Verification items for this drawing (mm, ordinates from the low corner). A direction names the side the tool comes from. Coordinates: 2 decimals unless noted, no trailing zeros. Write each loop counter-clockwise with the first axis right and the second up, starting at its lowest first coordinate (ties: lowest second). Pieces come first, ordered by that corner, then holes. Notation, with made-up numbers: (21.25, 66) -> (34.25, 66) arc R6 cw to (34.25, 70) -> close; hole circle Ø3 at (55, -7.5). An arc over 180 degrees is marked (long way). Answer as CSV lines item,"result".
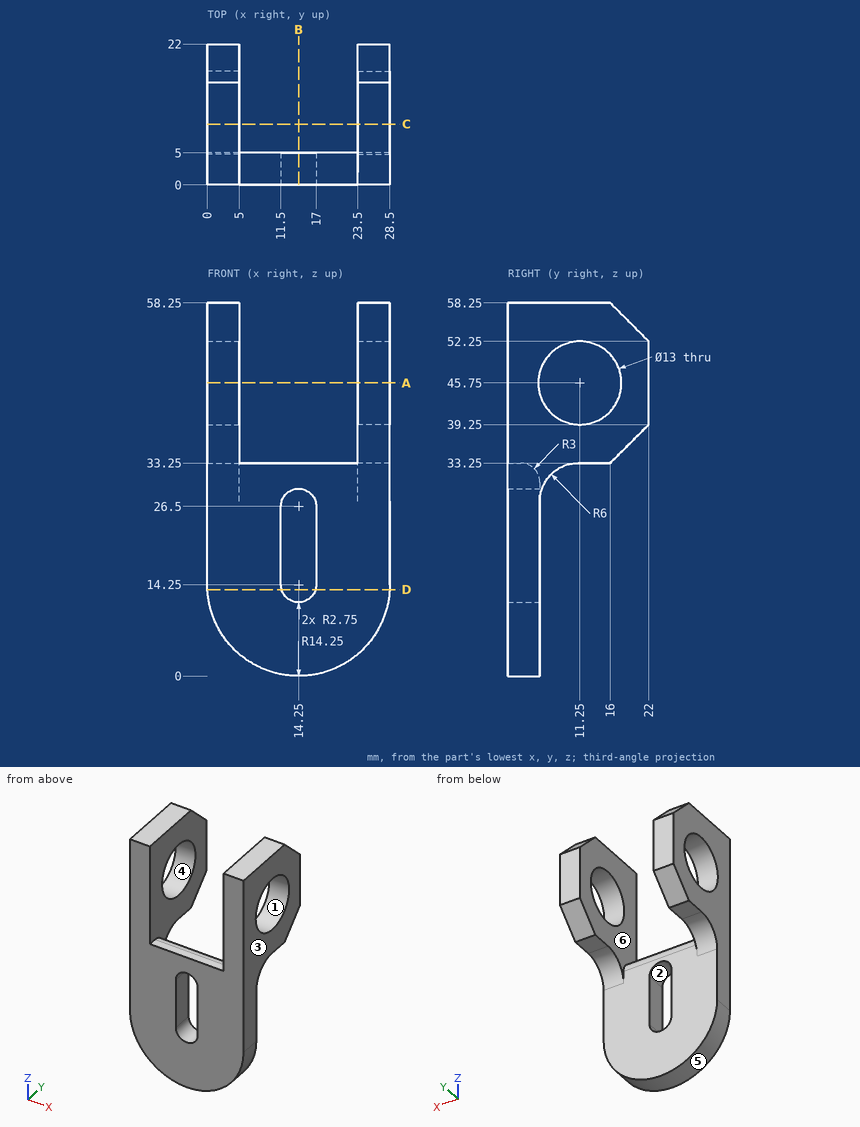
Item 1: Depth check by flat-ended pin: pin 1 Ø12 at (x, z) = (16.5, 7) entering from -Y; pin 2 Ø2 at (x, y) = (17, 0.5) entering from +Z; pin 3 Ø2.5 at (x, y) = (3, 14.5) entering from -Z; pin 4 Ø14 at (x, z) = (11, 22) entering from +Y. Enter the tip coordinate at first touch or a pass-through.
Responses:
pin 1,"stops at y = 0"
pin 2,"stops at z = 33.25"
pin 3,"stops at z = 33.25"
pin 4,"stops at y = 5"
Item 2: Set-up check for the marked faces 1 and 2: record each of +Z, -Z, +X, -X, +Y, -Y from which the full face is reachable in a straight line by a thin tool's end or side.
Responses:
face 1,"+X, -X"
face 2,"+Y, -Y"
Item 3: Cross-section at D-D, the plane z = 13.5. Record the cut outline in (x, y), plus the area to 3 significant figures.
Responses:
outline,"(0.02, 0) -> (11.6, 0) -> (11.6, 5) -> (0.02, 5) -> close; (16.9, 0) -> (28.48, 0) -> (28.48, 5) -> (16.9, 5) -> close"
area,"116 mm2"
Item 4: Cross-section at C-C, the plane y = 9.5. Record the cut outline in (x, z), plus the area to 3 significant figures.
Responses:
outline,"(0, 33.06) -> (5, 33.06) -> (5, 39.49) -> (0, 39.49) -> close; (0, 52.01) -> (5, 52.01) -> (5, 58.25) -> (0, 58.25) -> close; (23.5, 33.06) -> (28.5, 33.06) -> (28.5, 39.49) -> (23.5, 39.49) -> close; (23.5, 52.01) -> (28.5, 52.01) -> (28.5, 58.25) -> (23.5, 58.25) -> close"
area,"127 mm2"
Item 5: Release check for a two-part mould opening along X. For the marked faces 3, 4, 5 and 6 record: +X half, -X half, draft (parallel to the pull), parting line (faces both ways), or undercut.
Responses:
face 3,"+X half"
face 4,"draft"
face 5,"parting line"
face 6,"undercut"
Item 6: Thickness scan on probe 1 along X at (y, z) = (9.5, 33.5); probe 2 along Y at (x, z) = (25.4, 45.75); probe 3 along Z at (x, y) = (1.5, 8). Record the ranges inside material, lowest first.
Responses:
probe 1,"x = 0 to 5, 23.5 to 28.5"
probe 2,"y = 0 to 4.75, 17.75 to 22"
probe 3,"z = 32.45 to 40.12, 51.38 to 58.25"
Item 7: Cross-section at A-A, the plane z = 45.75. Record the cut outline in (x, y), plus the area to 3 significant figures.
Responses:
outline,"(0, 0) -> (5, 0) -> (5, 4.75) -> (0, 4.75) -> close; (0, 17.75) -> (5, 17.75) -> (5, 22) -> (0, 22) -> close; (23.5, 0) -> (28.5, 0) -> (28.5, 4.75) -> (23.5, 4.75) -> close; (23.5, 17.75) -> (28.5, 17.75) -> (28.5, 22) -> (23.5, 22) -> close"
area,"90.0 mm2"
Item 8: Cross-section at B-B, the plane x = 14.25. Record the cut outline in (y, z).
Responses:
outline,"(0, 0) -> (5, 0) -> (5, 11.5) -> (0, 11.5) -> close; (0, 29.25) -> (5, 29.25) -> (5, 30.25) arc R3 ccw to (2, 33.25) -> (0, 33.25) -> close"
